The model under review builds one solid part; all positions refer to its coordinate system, in mm. Face numbers are marked on the shaded views. A direction names the side the tool comes from. Coordinates: 2 decimals unless noted, no trailing zeros. Write each loop counter-clockwise with the first axis right and the second up, starting at its lowest first coordinate (ties: lowest second). Pieces come first, ordered by that corner, then holes. Notation, with made-up numbers: (55, 25.25) - (101, 25.25) arc R24 cw to (101, 57.25) - close; hole circle Ø4 at (76.5, -23.5). An arc over 180 degrees is marked (long way). Answer as CSV lines item,"result". Start each with the question number.
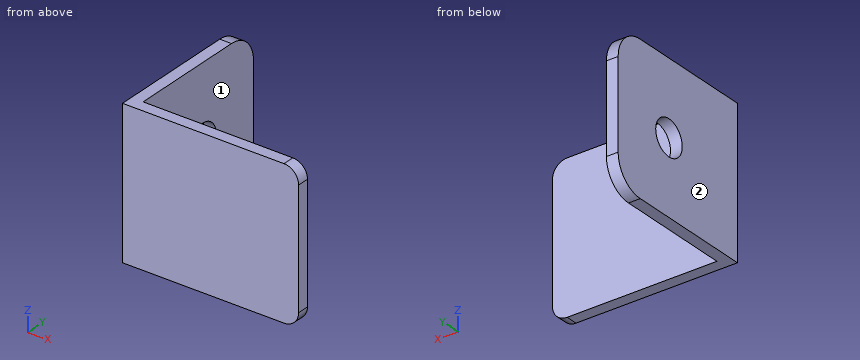
```python
from build123d import *

# Parameters (mm, degrees)
SKETCH1_W           = 60
SKETCH1_H           = 50
BOSS_EXTRUDE3_DEPTH = 4
SKETCH3_R           = 6
BOSS_EXTRUDE4_DEPTH = 4
FILLET1_R           = 5


with BuildPart() as part:
    # Sketch1 → Boss-Extrude3 (new body)
    with BuildSketch(Plane(origin=(0, 0, 0), x_dir=(1, 0, 0), z_dir=(0, 1, 0))):
        Rectangle(SKETCH1_W, SKETCH1_H)
    extrude(amount=BOSS_EXTRUDE3_DEPTH)

    # Sketch3 → Boss-Extrude4 (add)
    with BuildSketch(Plane.ZY.offset(30)):
        with BuildLine():
            Line((-25, 4), (25, 4))
            Line((25, 4), (25, 44))
            ThreePointArc((25, 44), (22.071067812, 51.071067812), (15, 54))
            Line((15, 54), (-15, 54))
            ThreePointArc((-15, 54), (-22.071067812, 51.071067812), (-25, 44))
            Line((-25, 44), (-25, 4))
        make_face()
        with Locations((0, 31)):
            Circle(SKETCH3_R, mode=Mode.SUBTRACT)
    extrude(amount=-BOSS_EXTRUDE4_DEPTH)

    # Fillet1
    fillet1_edges = [part.edges().sort_by_distance(p)[0] for p in [
        (30, 2, 25),
        (30, 2, -25),
    ]]
    fillet(fillet1_edges, radius=FILLET1_R)


solid = part.part
```
(1) For pin 1 (1 mm diameter, centred on x = 4, z = 4.5, fed in from +Y); pin 2 (25 mm diameter, centred on y = 41, z = 3, fed in from +X); pin 3 (1 mm diameter, centred on y = 28.5, z = 3.5, fed in from +X), all flat-tipped, find the tip position at first contact; note any pin that passes through.
(2) Add section A-A on y = 31. Give the boundary of the cut face in (x, z).
(3) Add section B-B on z = 5. Give the boundary of the cut face in (x, y).
(4) For the marked faces 1 and 2, list the 3-axis set-ups (+Z, -Z, +X, -X, +Y, -Y) from which the entire face can be reached by the end or side of a thin tool; tool diameter is ignored.
(5) Wall thickness on line 1 (Y direction, x = -27.4, z = 0); line 2 (Y direction, x = 27.5, z = 3.5); line 3 (X direction, y = 28.5, z = -14): over which ranges is each line inside the solid? List them lowest first.
(6) Add section D-D on z = 0. Give the boundary of the cut face in (x, y).
(7) Add section C-C on x = -19. Give the boundary of the cut face in (y, z), then the cut area to 3 significant figures.
Reported:
1,pin 1,"y = 4"
1,pin 2,"x = -26"
1,pin 3,"through"
2,outline,"(-30, -25) - (-26, -25) - (-26, -6) - (-30, -6) - close; (-30, 6) - (-26, 6) - (-26, 25) - (-30, 25) - close"
3,outline,"(-30, 0) - (30, 0) - (30, 4) - (-26, 4) - (-26, 27.68) - (-30, 27.68) - close; (-30, 34.32) - (-26, 34.32) - (-26, 54) - (-30, 54) - close"
4,face 1,"+Z, -Z, +X, +Y"
4,face 2,"+Z, -Z, -X, +Y, -Y"
5,line 1,"0 to 25, 37 to 54"
5,line 2,"0 to 4"
5,line 3,"-30 to -26"
6,outline,"(-30, 0) - (30, 0) - (30, 4) - (-26, 4) - (-26, 25) - (-30, 25) - close; (-30, 37) - (-26, 37) - (-26, 54) - (-30, 54) - close"
7,outline,"(0, -25) - (4, -25) - (4, 25) - (0, 25) - close"
7,area,"200 mm²"
